Geometry: final body of the model. Coordinates: model frame, mm. Face numbers are marked on the shaded views. A direction names the side the tool comes from. Give positions to 0.01 mm unless a question says otherwise; leave off trailing zeros. Write each loop counter-clockwise with the first axis right and the second up, starting at its lowest first coordinate (ties: lowest second). Pieces come first, ordered by that corner, then holes.
Q1. Line query: L1, parallel to X at y = 18.85, z = 17.5; L2, parallel to Y at x = 5.5, z = -2; L3, parallel to Z at x = 14, y = 18.5. Output: solid intervals per line, ascending.
Q2. Cut plane D-D on x = -8. Return the cut outline in (y, z), plus the area to 3 significant figures.
Q3. Cut plane C-C on y = 17.75. Return the cut outline in (x, z), plus the area to 3 significant figures.
Q4. Cut plane B-B on z = 0. Return the cut outline in (x, y), plus the area to 3 significant figures.
Q5. Pin query (flat end, axial travel): pin 1 (5.5 mm diameter, centred on x = 0, z = -17.5, fed in from +Y); pin 2 (10 mm diameter, centred on y = 11.5, z = -5.5, fed in from -X); pin 3 (4.5 mm diameter, centred on y = 27, z = 0, fed in from -X). Return the tip coordinate at first contact, or that it passes through.
Q6. Cut plane A-A on x = 0. Return the cut outline in (y, z).
Q7. Reachability of the marked faces 1, 2, 3 and 4 from +Z, -Z, +X, -X, +Y, -Y: full face, straight path, thin tool, end or side. Return the list, or none.
```python
from build123d import *

# Parameters (mm, degrees)
BOSS_EXTRUDE1_DEPTH = 19
SKETCH3_R           = 2.1
BOSS_EXTRUDE2_DEPTH = 0.5
SKETCH4_R           = 4.5
BOSS_EXTRUDE3_DEPTH = 1.5
SKETCH5_R           = 2.5
BOSS_EXTRUDE4_DEPTH = 8.5
CUT_EXTRUDE1_START  = -6
CUT_EXTRUDE1_DEPTH  = 6


with BuildPart() as part:
    # Sketch1 → Boss-Extrude1 (new body)
    with BuildSketch(Plane(origin=(0, 0, 0), x_dir=(1, 0, 0), z_dir=(0, 1, 0))):
        with BuildLine():
            Line((11.94612908, 7.3), (17, 7.3))
            Line((17, 7.3), (17, -7.3))
            Line((17, -7.3), (11.94612908, -7.3))
            ThreePointArc((11.94612908, -7.3), (-14, 0), (11.94612908, 7.3))
        make_face()
    extrude(amount=BOSS_EXTRUDE1_DEPTH)

    # Sketch3 → Boss-Extrude2 (add)
    with BuildSketch(Plane(origin=(0, 19, 0), x_dir=(1, 0, 0), z_dir=(0, 1, 0))):
        with BuildLine():
            Line((3.5, 17.5), (3.5, -17.5))
            ThreePointArc((3.5, -17.5), (0, -21), (-3.5, -17.5))
            Line((-3.5, -17.5), (-3.5, 17.5))
            ThreePointArc((-3.5, 17.5), (0, 21), (3.5, 17.5))
        make_face()
        with Locations(Location((0, -17.5, 0), (0, 0, 270))):
            Circle(SKETCH3_R, mode=Mode.SUBTRACT)
        with Locations(Location((0, 17.5, 0), (0, 0, 270))):
            Circle(SKETCH3_R, mode=Mode.SUBTRACT)
    extrude(amount=-BOSS_EXTRUDE2_DEPTH)

    # Sketch4 → Boss-Extrude3 (add)
    with BuildSketch(Plane(origin=(0, 19, 0), x_dir=(1, 0, 0), z_dir=(0, 1, 0))):
        with Locations(Location((-8, 0, 0), (0, 0, 270))):
            Circle(SKETCH4_R)
    extrude(amount=BOSS_EXTRUDE3_DEPTH)

    # Sketch5 → Boss-Extrude4 (add)
    with BuildSketch(Plane(origin=(0, 20.5, 0), x_dir=(1, 0, 0), z_dir=(0, 1, 0))):
        with Locations(Location((-8, 0, 0), (0, 0, 270))):
            Circle(SKETCH5_R)
    extrude(amount=BOSS_EXTRUDE4_DEPTH)

    # Sketch6 → Cut-Extrude1 (cut)
    with BuildSketch(Plane(origin=(0, 29, 0), x_dir=(1, 0, 0), z_dir=(0, 1, 0)).offset(CUT_EXTRUDE1_START)):
        with BuildLine():
            Line((-9.5, 2), (-9.5, -2))
            ThreePointArc((-9.5, -2), (-10.5, 0), (-9.5, 2))
        make_face()
        with BuildLine():
            Line((-6.5, 2), (-6.5, -2))
            ThreePointArc((-6.5, -2), (-5.5, 0), (-6.5, 2))
        make_face()
    extrude(amount=CUT_EXTRUDE1_DEPTH, mode=Mode.SUBTRACT)


solid = part.part
```
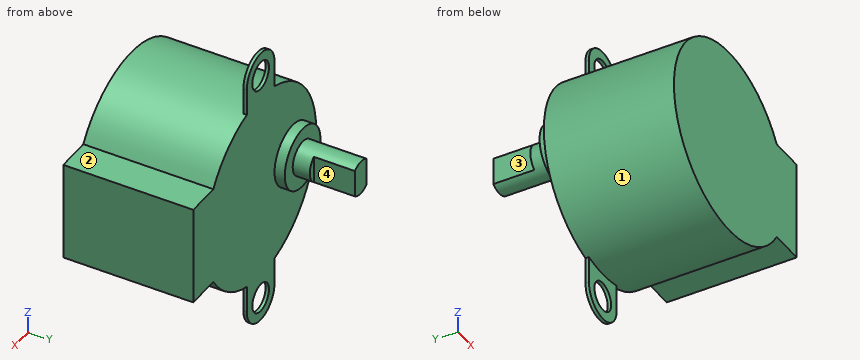
Data:
1. L1: x = -3.5 to -2.1, 2.1 to 3.5
1. L2: y = 0 to 19
1. L3: z = -7.3 to 7.3
2. outline: (0, -11.49) - (19, -11.49) - (19, -4.5) - (20.5, -4.5) - (20.5, -2.5) - (29, -2.5) - (29, 2.5) - (20.5, 2.5) - (20.5, 4.5) - (19, 4.5) - (19, 11.49) - (0, 11.49) - close
2. area: 493 mm2
3. outline: (11.95, -7.3) - (17, -7.3) - (17, 7.3) - (11.95, 7.3) arc R14 ccw (long way) to start
3. area: 669 mm2
4. outline: (-14, 0) - (17, 0) - (17, 19) - (-3.5, 19) - (-3.5, 20.5) - (-5.5, 20.5) - (-5.5, 23) - (-6.5, 23) - (-6.5, 29) - (-9.5, 29) - (-9.5, 23) - (-10.5, 23) - (-10.5, 20.5) - (-12.5, 20.5) - (-12.5, 19) - (-14, 19) - close
4. area: 633 mm2
5. pin 1: stops at y = 19
5. pin 2: stops at x = -13.99
5. pin 3: stops at x = -9.5
6. outline: (0, -14) - (18.5, -14) - (18.5, -15.4) - (19, -15.4) - (19, 15.4) - (18.5, 15.4) - (18.5, 14) - (0, 14) - close; (18.5, -21) - (19, -21) - (19, -19.6) - (18.5, -19.6) - close; (18.5, 19.6) - (19, 19.6) - (19, 21) - (18.5, 21) - close
7. face 1: -Y
7. face 2: +Z, +X, +Y, -Y
7. face 3: +Z, -Z, -X, +Y
7. face 4: +Z, -Z, +X, +Y
